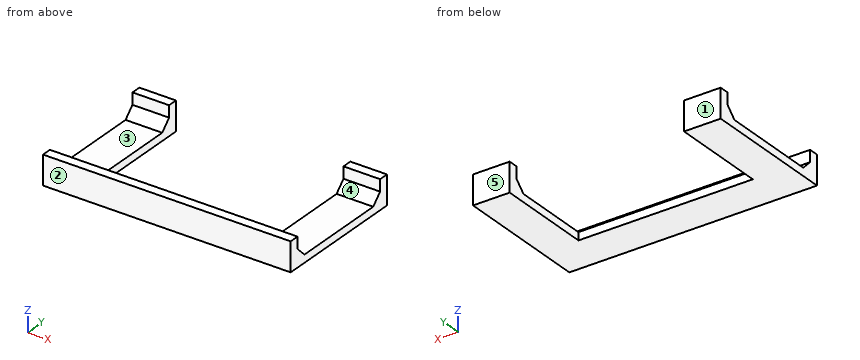
from build123d import *

# Parameters (mm, degrees)
F0_W     = 127.826088
F0_H     = 5
F0_W_2   = 18.913044
F1_DEPTH = 4
F2_DEPTH = 15
F3_SIZE  = 5


with BuildPart() as f1:
    # F0 (on Top) → F1 (new body)
    with BuildSketch(Plane.XY):
        Polygon((-25.108697, 38.340694), (-44.021741, 38.340694), (-44.021741, -21.659306), (83.804347, -21.659306), (83.804347, 38.340694), (64.891303, 38.340694), (64.891303, -6.659306), (-25.108697, -6.659306), align=None)
        with Locations((19.891303, -24.159306)):
            Rectangle(F0_W, F0_H)
        with Locations((-34.565219, 40.840694)):
            Rectangle(F0_W_2, F0_H)
    extrude(amount=F1_DEPTH)

    # F0 (on Top) → F2 (join)
    with BuildSketch(Plane.XY):
        with Locations((19.891303, -24.159306)):
            Rectangle(F0_W, F0_H)
        with Locations((-34.565219, 40.840694)):
            Rectangle(F0_W_2, F0_H)
        with Locations((74.347825, 40.840694)):
            Rectangle(F0_W_2, F0_H)
    extrude(amount=F2_DEPTH)

    # F3
    f3_edges = [f1.edges().sort_by_distance(p)[0] for p in [
        (19.891303, -21.659306, 4),
        (-34.565219, 38.340694, 4),
        (74.347825, 38.340694, 4),
    ]]
    chamfer(f3_edges, length=F3_SIZE)


solid = f1.part
Can you work these out from the model? Positions are in its coordinate system, mm. Face numbers are marked on the shaded views. A direction names the side the tool comes from. Round coordinates to 2 decimals unless told otherwise and drop trailing zeros. Order: outer loops, then holes, each group sorted by start corner. A loop starts at its lowest first (then second) coordinate and runs counter-clockwise, first axis right, second up. Notation, with made-up numbers: (-34.75, -17.5) - (-11.75, -17.5) arc R26 cw to (-11.75, -2.5) - close; hole circle Ø8 at (47, 20). An arc over 180 degrees is marked (long way). Answer in a Markdown table with one row per item.
(1) Suppose I cut it at A-A, the plane z = 10.5. Please give me the cut outline in (x, y).
From the geometry:
| item | result |
|---|---|
| outline | (-44.02, -26.66) - (83.8, -26.66) - (83.8, -21.66) - (-44.02, -21.66) - close; (-44.02, 38.34) - (-25.11, 38.34) - (-25.11, 43.34) - (-44.02, 43.34) - close; (64.89, 38.34) - (83.8, 38.34) - (83.8, 43.34) - (64.89, 43.34) - close |
(2) Please list where these lines run through material, in increasing order: L1, parallel to Y at x = 74.5, z = 9.75; L2, parallel to X at y = 0, z = 3.25; L3, parallel to Z at x = -2.5, y = -16. Write a range as from..to.
From the geometry:
| item | result |
|---|---|
| L1 | y = -26.66..-21.66, 38.34..43.34 |
| L2 | x = -44.02..-25.11, 64.89..83.8 |
| L3 | z = 0..4 |
(3) If we mould it in two halves opening along Y, with no side actions, what happens to the marked faces 1, 2 and 3? For each: released by +Y, released by -Y, zero draft, split by the parting line, or undercut.
From the geometry:
| item | result |
|---|---|
| face 1 | released by +Y |
| face 2 | released by -Y |
| face 3 | undercut |
(4) For P1, Ø15, axis at x = 10, y = 0, coming from the +Z side; P2, Ø1.5, axis at x = 39, z = 10, coming from the +Y side; P3, Ø7.5, axis at y = 16, z = 10, coming from the +X side; P4, Ø3, axis at x = 23.5, z = 2, coming from the +Y side, each with a flat end and sliding along its axis, tell me the tip position at first contact or that it passes through.
From the geometry:
| item | result |
|---|---|
| P1 | stops at z = 4 |
| P2 | stops at y = -21.66 |
| P3 | passes through |
| P4 | stops at y = -6.66 |
(5) Suppose I cut it at D-D, the plane y = -10.5. Please give me the cut outline in (x, z).
From the geometry:
| item | result |
|---|---|
| outline | (-44.02, 0) - (83.8, 0) - (83.8, 4) - (-44.02, 4) - close |
(6) Which directions (+Z, -Z, +X, -X, +Y, -Y) give clear straight access to the entire face, cutting with the end or side of a thin tool? Please do the marked faces 4 and 5.
From the geometry:
| item | result |
|---|---|
| face 4 | +Z, +X, -X |
| face 5 | +Z, -Z, +X, -X, +Y |
(7) Suppose I cut it at C-C, the plane x = -29. Please give me the cut outline in (y, z).
From the geometry:
| item | result |
|---|---|
| outline | (-26.66, 0) - (43.34, 0) - (43.34, 15) - (38.34, 15) - (38.34, 9) - (33.34, 4) - (-16.66, 4) - (-21.66, 9) - (-21.66, 15) - (-26.66, 15) - close |
(8) Suppose I cut it at B-B, the plane y = 12. Please give me the cut outline in (x, z), plus the area to 3 significant figures.
From the geometry:
| item | result |
|---|---|
| outline | (-44.02, 0) - (-25.11, 0) - (-25.11, 4) - (-44.02, 4) - close; (64.89, 0) - (83.8, 0) - (83.8, 4) - (64.89, 4) - close |
| area | 151 mm2 |
